Autodesk Fusion 360 part; units mm, degrees
sketch "Sketch1" plane through (0, 0, 0) normal (0, 0, 1) x (1, 0, 0)
  circle A0 centre (0, 0) radius 60
  circle A1 centre (0, 0) radius 58
  circle A2 centre (0, 0) radius 60.5
  circle A3 centre (0, 0) radius 62.5
  dimension "d1" = 120
  dimension "d2" = 116
  dimension "d3" = 121
  dimension "d4" = 125
extrude "Extrude1" add sketch "Sketch1" along normal blind 20 makes body 1 at (59.9254, -2.9908, 13.3333) makes body 2 at (62.4223, -3.1154, 13.3333)
sketch "Sketch2" plane through (0, 0, 0) normal (0, 0, -1) x (1, 0, 0)
  circle A0 centre (0, 0) radius 58
  circle A1 centre (0, 0) radius 60
  circle A2 centre (0, 0) radius 60
  circle A3 centre (0, 0) radius 60.5
  dimension "d11" = 120
  dimension "d12" = 121
extrude "Extrude2" add sketch "Sketch1" against normal blind 4 contours A0 | A2 | A3 bodies 2 1
sketch "Sketch3" plane through (0, 0, -4) normal (0, 0, -1) x (1, 0, 0)
  circle A0 centre (0, 0) radius 58
  circle A1 centre (0, 0) radius 62.5
  circle A2 centre (0, 0) radius 58
  circle A3 centre (0, 0) radius 60
  circle A4 centre (0, 0) radius 60.5
  circle A5 centre (0, 0) radius 62.5
  dimension "d13" = 116
  dimension "d14" = 120
  dimension "d15" = 121
  dimension "d16" = 125
extrude "Extrude4" add sketch "Sketch3" along normal blind 20 bodies 2
sketch "Sketch4" plane through (0, 0, 20) normal (0, 0, 1) x (-1, 0, 0)
  circle A0 centre (0, 0) radius 60.5
  circle A1 centre (0, 0) radius 62.5
  line L0 (0, 0) -> (0, 62.5)
  line L1 (0, 0) -> (-20.5, 0)
  line L2 (0, 62.5) -> (20.5, 62.5)
  line L3 (-20.5, 0) -> (20.5, 0)
  line L4 (20.5, 0) -> (20.5, 62.5)
  line L5 (20.5, 62.5) -> (-20.5, 62.5)
  line L6 (-20.5, 62.5) -> (-20.5, 0)
  circle A2 centre (0, 0) radius 60
  dimension "d19" = 20.5
  dimension "d21" = 20.5
  dimension "d22" = 120
extrude "Extrude5" add sketch "Sketch4" against normal blind 20 contours A0 L0 L4 A2 | A0 L0 L6 A2 bodies 2
copy_body "Body->Comp1" bodies 2 removing the originals makes body 3 in component "midjoint"
sketch "Sketch5" plane through (0, 0, -24) normal (0, 0, -1) x (1, 0, 0)
  circle A0 centre (0, 0) radius 58
  circle A1 centre (0, 0) radius 60
  circle A2 centre (0, 0) radius 59.25
  circle A3 centre (0, 0) radius 61.25
  dimension "d35" = 118.5
  dimension "d36" = 122.5
extrude "Extrude1'" cut sketch "Sketch5" against normal blind 20 contours A1 | A3 bodies 3 in component "midjoint"
sketch "Sketch6" plane through (0, 0, 20) normal (0, 0, 1) x (-1, 0, 0)
  circle A0 centre (0, 0) radius 62.5
  circle A1 centre (0, 0) radius 58
  arc A2 (-20.5, 56.3893) -> (20.5, 56.3893) centre (0, 0) ccw
  line L0 (20.5, 56.3893) -> (20.5, 56.921)
  arc A3 (-20.5, 56.921) -> (20.5, 56.921) centre (0, 0) ccw
  line L1 (-20.5, 56.921) -> (-20.5, 56.3893)
  circle A4 centre (0, 0) radius 59.25
  circle A5 centre (-0.0055, -0.0156) radius 61.25
  line L2 (20.5, 56.921) -> (20.5, 57.7)
  line L3 (20.5, 56.3893) -> (20.5, 55.5906)
  line L4 (-20.5, 56.921) -> (-20.5, 57.7039)
  line L5 (-20.5, 56.3893) -> (-20.5, 55.5906)
  dimension "d33" = 118.5
  dimension "d34" = 122.5
extrude "Extrude2'" cut sketch "Sketch6" against normal blind 20 contours A2 A4 L3 L5 | A2 L0 A3 L1 | A3 A5 L2 L4 bodies 3 in component "midjoint"
component "midjoint" placed x (1, 0, 0) y (0, 1, 0) z (0, 0, 1) at (0, 0, 0)
Work out the finished part from the listing and answer in its coordinate system (mm). A direction names the side the tool comes from. Give positions to 0.01 mm unless a question says otherwise; leave off trailing zeros. Loops run counter-clockwise (first coordinate to the right, second up) from the corner with the lowest first, then second, coordinate; pieces in that order, holes last. Notation, with made-up numbers: (-19, 64.25) - (0, 64.25) arc R16 cw to (0, 84.25) - close; hole circle Ø5 at (61.5, 74.25). An arc over 180 degrees is marked (long way). Answer in a Markdown table with one row per item.
(1) For a pull along X with two mould halves and no side action, classify faces 4 (the face through (44, 39, -24)), 5 (the face through (-13.278, 59.793, -14.14)), 6 (the face through (-62.44, 2.75, -1.69)) as pulls with the +X half, pulls with the -X half, needs draft (parallel to the pull), parting line crosses it, or undercut.
Results list:
| item | result |
|---|---|
| face 4 | needs draft |
| face 5 | undercut |
| face 6 | parting line crosses it |
(2) Flat-ended cylindrical pins translate along their axes: pin 1 Ø4 at (y, z) = (10.5, -9.5) entering from -X; pin 2 Ø8 at (y, z) = (13.5, -15) entering from -X; pin 3 Ø10 at (y, z) = (48.5, -2.5) entering from -X. Find the tip coordinate at first contact, or state that the pin passes through.
Results list:
| item | result |
|---|---|
| pin 1 | stops at x = -61.92 |
| pin 2 | stops at x = -61.77 |
| pin 3 | stops at x = -44.88 |
(3) Consider L1, parallel to X at y = -0.5, z = -15.5; L2, parallel to Y at x = -23, z = 2.5. Determine where each line is inside the solid, lowest interval first. Write a range as [from, to].
Results list:
| item | result |
|---|---|
| L1 | x = [-62.5, -61.25], [-59.25, -58], [58, 59.25], [61.25, 62.5] |
| L2 | y = [-58.11, -56.75], [-54.6, -53.24], [53.24, 54.6], [56.78, 58.11] |
(4) Section A-A (y = 0) is taken. Give the vertices of the cut face in (x, z), and give its area (3 significant figures).
Results list:
| item | result |
|---|---|
| outline | (-62.5, -24) - (-61.25, -24) - (-61.25, -4) - (-59.25, -4) - (-59.25, -24) - (-58, -24) - (-58, 20) - (-59.25, 20) - (-59.25, 0) - (-61.24, 0) - (-61.24, 20) - (-62.5, 20) - close; (58, -24) - (59.25, -24) - (59.25, -4) - (61.25, -4) - (61.25, -24) - (62.5, -24) - (62.5, 20) - (61.26, 20) - (61.26, 0) - (59.25, 0) - (59.25, 20) - (58, 20) - close |
| area | 236 mm² |
(5) Section D-D (y = -53) is taken. Give the vertices of the cut face in (x, z).
Results list:
| item | result |
|---|---|
| outline | (-33.12, -24) - (-30.7, -24) - (-30.7, -4) - (-26.49, -4) - (-26.49, -24) - (-23.56, -24) - (-23.56, 20) - (-26.49, 20) - (-26.49, 0) - (-30.67, 0) - (-30.67, 20) - (-33.12, 20) - close; (23.56, -24) - (26.49, -24) - (26.49, -4) - (30.7, -4) - (30.7, -24) - (33.12, -24) - (33.12, 20) - (30.68, 20) - (30.68, 0) - (26.49, 0) - (26.49, 20) - (23.56, 20) - close |
(6) Section C-C (z = -20.5) is taken. Give the vertices of the cut face in (x, y), and give its area (3 significant figures).
Results list:
| item | result |
|---|---|
| outline | circle Ø125 at (0, 0); circle Ø118.5 at (0, 0); hole circle Ø122.5 at (0, 0); hole circle Ø116 at (0, 0) |
| area | 946 mm² |
(7) Section B-B (x = 0) is taken. Give the vertices of the cut face in (y, z).
Results list:
| item | result |
|---|---|
| outline | (-62.5, -24) - (-61.25, -24) - (-61.25, -4) - (-59.25, -4) - (-59.25, -24) - (-58, -24) - (-58, 20) - (-62.5, 20) - close; (58, -24) - (59.25, -24) - (59.25, -4) - (61.25, -4) - (61.25, -24) - (62.5, -24) - (62.5, 20) - (61.27, 20) - (61.27, 0) - (59.25, 0) - (59.25, 20) - (58, 20) - close |
(8) A tool of negligible diameter and unlimited length cuts with its end or side. For faces 1 (the face through (-4.8, 59.3, 0)), 2 (the face through (46, 41, -24)), 3 (the face through (-32, -50.2, -4)), from which of +Z, -Z, +X, -X, +Y, -Y can it reach the whole face along a straight path? Write none if from no direction.
Results list:
| item | result |
|---|---|
| face 1 | +Z |
| face 2 | -Z, +X, -X, +Y, -Y |
| face 3 | -Z |
